```python
from build123d import *

# Parameters (mm, degrees)
SKETCH1_W               = 260
SKETCH1_H               = 30
BOSS_EXTRUDE1_DEPTH     = 40
ESQUISSE1_R             = 2
ENL_V_MAT_EXTRU_1_DEPTH = 265.764045897
ESQUISSE2_R             = 3
ENL_V_MAT_EXTRU_2_DEPTH = 265.764045897


with BuildPart() as part:
    # Sketch1 → Boss-Extrude1 (new body)
    with BuildSketch(Plane.XY):
        with Locations((130, 15)):
            Rectangle(SKETCH1_W, SKETCH1_H)
    extrude(amount=BOSS_EXTRUDE1_DEPTH)

    # Esquisse1 → Enlèv. mat.-Extru.1 (cut, through all)
    with BuildSketch(Plane.XY.offset(40)):
        with Locations((7, 22)):
            Circle(ESQUISSE1_R)
        with Locations((37, 22)):
            Circle(ESQUISSE1_R)
    extrude(amount=-ENL_V_MAT_EXTRU_1_DEPTH, mode=Mode.SUBTRACT)

    # Esquisse2 → Enlèv. mat.-Extru.2 (cut, through all)
    with BuildSketch(Plane(origin=(260, 0, 0), x_dir=(0, 0, -1), z_dir=(1, 0, 0))):
        with Locations((-10, 8)):
            Circle(ESQUISSE2_R)
        with Locations((-30, 8)):
            Circle(ESQUISSE2_R)
    extrude(amount=-ENL_V_MAT_EXTRU_2_DEPTH, mode=Mode.SUBTRACT)


solid = part.part
```
Geometry check sheet. Reference: the model listing, model coordinates, mm. Coordinates: 2 decimals unless noted, no trailing zeros. Loops run counter-clockwise (first coordinate to the right, second up) from the corner with the lowest first, then second, coordinate; pieces in that order, holes last. Notation, with made-up numbers: (40.5, 55.25) - (77.5, 55.25) arc R21 cw to (77.5, 78.25) - close; hole circle Ø4 at (-29, -16). An arc over 180 degrees is marked (long way). One line per item, written item: value. Start each with the question number.
(1) Cross-section at B-B on x = 127. Enter the section's corners in (y, z).
(2) Material ranges on line 1 (Y direction, x = 143, z = 30); line 2 (Z direction, x = 164.5, y = 10.25); line 3 (Y direction, x = 37, z = 24.5), recorded low to high. Write a range as [from, to].
(3) Cross-section at A-A on z = 30. Enter the section's corners in (x, y), plus the area to 3 significant figures.
(4) Mould release check, pull along X, two halves, no side actions. Record for faces 1 (the cylindrical face through (5.4, 20.8, 20.3)), 2 (the flat face through (260, 15, 20)), 3 (the flat face through (128, 15, 0)): released by +X, released by -X, zero draft, split by the parting line, or undercut.
Results below:
1. outline: (0, 0) - (30, 0) - (30, 40) - (0, 40) - close; hole circle Ø6 at (8, 10); hole circle Ø6 at (8, 30)
2. line 1: y = [0, 5], [11, 30]
2. line 2: z = [0, 8.02], [11.98, 28.02], [31.98, 40]
2. line 3: y = [0, 20], [24, 30]
3. outline: (0, 0) - (260, 0) - (260, 5) - (0, 5) - close; (0, 11) - (260, 11) - (260, 30) - (0, 30) - close; hole circle Ø4 at (7, 22); hole circle Ø4 at (37, 22)
3. area: 6,210 mm2
4. face 1: undercut
4. face 2: released by +X
4. face 3: zero draft
